The model under review builds one solid part; all positions refer to its coordinate system, in mm. Face numbers are marked on the shaded views. A direction names the side the tool comes from. Coordinates: 2 decimals unless noted, no trailing zeros. Write each question's results on one line, items separated by ' | '.
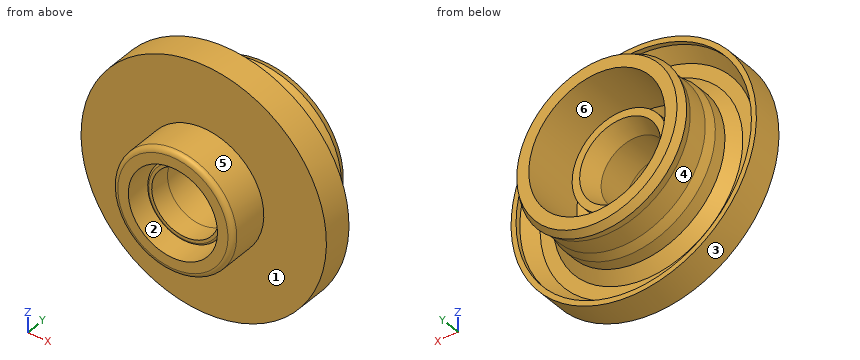
```python
from build123d import *

# Parameters (mm, degrees)
SKETCH8_R           = 3.85
SKETCH8_R_2         = 3.35
BOSS_EXTRUDE1_DEPTH = 2.1
FILLET2_R           = 0.5
FILLET3_R           = 0.2


with BuildPart() as part:
    # Sketch1 → Revolve1 (revolve)
    with BuildSketch(Plane.XY, mode=Mode.PRIVATE) as revolve1_sk:
        Polygon((-12.25, 7.1), (-4.45, 7.1), (-4.45, 0), (-6, 0), (-6, 4.1), (-12.25, 4.1), align=None)
    revolve(revolve1_sk.sketch.rotate(Axis((0, 0, 0), (0, 1, 0)), 270), axis=Axis((0, 0, 0), (0, 1, 0)))

    # Sketch6 → Cut-Revolve2 (revolve, cut)
    with BuildSketch(Plane.XY, mode=Mode.PRIVATE) as cut_revolve2_sk:
        Polygon((-11.75, 7.1), (-11.75, 6.6), (-10.769709447, 5.2), (-6.8, 5.2), (-6.8, 4.5), (0, 4.5), (0, 7.1), (0, 9.850026385), (-11.75, 9.850026385), align=None)
    revolve(cut_revolve2_sk.sketch.rotate(Axis((0, 4.5, 0), (0, 1, 0)), 270), axis=Axis((0, 4.5, 0), (0, 1, 0)), mode=Mode.SUBTRACT)

    # Sketch7 → Revolve2 (revolve)
    with BuildSketch(Plane.XY, mode=Mode.PRIVATE) as revolve2_sk:
        Polygon((-4.8, 8.9), (-4.8, 3.744419371), (-3.35, 3.744419371), (-3.35, 6.976765806), (-4.05, 8.9), align=None)
    revolve(revolve2_sk.sketch.rotate(Axis((0, 0, 0), (0, 1, 0)), 270), axis=Axis((0, 0, 0), (0, 1, 0)))

    # Sketch8 → Boss-Extrude1 (add)
    with BuildSketch(Plane.XZ.offset(-3.744419371)):
        with Locations(Location((0, 0, 0), (0, 0, 90))):
            Circle(SKETCH8_R)
        with Locations(Location((0, 0, 0), (0, 0, 270))):
            Circle(SKETCH8_R_2, mode=Mode.SUBTRACT)
    extrude(amount=BOSS_EXTRUDE1_DEPTH)

    # Sketch9 → Revolve3 (revolve)
    with BuildSketch(Plane.XY, mode=Mode.PRIVATE) as revolve3_sk:
        Polygon((-6.799806645, 12), (-6.799806645, 5.2), (-9.469806645, 5.2), (-8.45, 6.219806645), (-8.45, 7.5), (-8.2, 8.5), (-8.2, 10.5), (-8.400961894, 11.25), (-7.999806645, 12), align=None)
    revolve(revolve3_sk.sketch.rotate(Axis((0, 0, 0), (0, 1, 0)), 270), axis=Axis((0, 0, 0), (0, 1, 0)))

    # Sketch11 → Revolve4 (revolve)
    with BuildSketch(Plane.XY, mode=Mode.PRIVATE) as revolve4_sk:
        Polygon((-6.799806645, 5.6), (-6, 4.5), (-6, 4.308890283), (-7.13977868, 4.308890283), (-7.13977868, 5.6), align=None)
    revolve(revolve4_sk.sketch.rotate(Axis((0, 0, 0), (0, 1, 0)), 270), axis=Axis((0, 0, 0), (0, 1, 0)))

    # Fillet2
    fillet2_edges = [part.edges().sort_by_distance(p)[0] for p in [
        (0, 0, 6),
    ]]
    fillet(fillet2_edges, radius=FILLET2_R)

    # Fillet3
    fillet3_edges = [part.edges().sort_by_distance(p)[0] for p in [
        (0, 1.644419371, -3.85),
    ]]
    fillet(fillet3_edges, radius=FILLET3_R)


solid = part.part
```
Q1. For line 1 (X direction, y = 2.4, z = 0); line 2 (X direction, y = 6.25, z = -1.5); line 3 (Z direction, x = -0.75, y = 8.25), list the stretches that pass through material, from the lowest coordinate up. Write a range as from..to.
Solution:
line 1: -6..-4.45, -3.85..-3.35, 3.35..3.85, 4.45..6 | line 2: -12.16..-11.41, -8.32..-6.63, -4.56..-3, 3..4.56, 6.63..8.32, 11.41..12.16 | line 3: -8.23..-6.76, -4.74..-3.74, 3.74..4.74, 6.76..8.23
Q2. Machinability: for the marked faces 4, 5 and 6, which of the approach directions +Z, -Z, +X, -X, +Y, -Y give a long, thin tool a straight path to every point of the face, cutting with its end or side? Answer none if there is none.
Solution:
face 4: none | face 5: -Y | face 6: +Y
Q3. Clearance check with flat-ended pins moving along their axes: P1, Ø5, axis at y = 11, z = 1.5, coming from the -X side; P2, Ø1, axis at x = -9.5, z = -9, coming from the -Y side; P3, Ø3.5, axis at x = -1.5, z = 1.5, coming from the -Y side; P4, Ø1, axis at x = -2.5, y = 1.5, coming from the -Z side. State where each tip first meets the part, or that it passes through.
Solution:
P1: x = -8.4 | P2: through | P3: y = 1.64 | P4: z = -5.66
Q4. Draft analysis for pull direction X (two halves, no side actions). For the marked faces 1, 2 and 3, state which applies: pulls with the +X half, pulls with the -X half, needs draft (parallel to the pull), parting line crosses it, or undercut.
Solution:
face 1: needs draft | face 2: undercut | face 3: parting line crosses it
